```python
from build123d import *

# Parameters (mm, degrees)
BOSS_EXTRUDE1_DEPTH = 1.5
BOSS_EXTRUDE2_DEPTH = 3


with BuildPart() as part:
    # Sketch3 → Boss-Extrude1 (new body)
    with BuildSketch(Plane.XY):
        with BuildLine():
            Line((-20, 0), (-20, -97))
            ThreePointArc((-20, -97), (0, -117), (20, -97))
            Line((20, -97), (20, 0))
            ThreePointArc((20, 0), (0, 20), (-20, 0))
        make_face()
    extrude(amount=BOSS_EXTRUDE1_DEPTH)

    # Sketch5 → Boss-Extrude2 (add)
    with BuildSketch(Plane.XY.offset(1.5)):
        with BuildLine():
            Line((-19, 0), (-19, -97))
            ThreePointArc((-19, -97), (0, -116), (19, -97))
            Line((19, -97), (19, 0))
            ThreePointArc((19, 0), (0, 19), (-19, 0))
        make_face()
        with BuildLine():
            Line((-18, 0), (-18, -97))
            ThreePointArc((-18, -97), (0, -115), (18, -97))
            Line((18, -97), (18, 0))
            ThreePointArc((18, 0), (0, 18), (-18, 0))
        make_face(mode=Mode.SUBTRACT)
    extrude(amount=BOSS_EXTRUDE2_DEPTH)


solid = part.part
```
Work out the finished part from the listing and answer in its coordinate system (mm). A direction names the side the tool comes from. Coordinates: 2 decimals unless noted, no trailing zeros. Loops run counter-clockwise (first coordinate to the right, second up) from the corner with the lowest first, then second, coordinate; pieces in that order, holes last.
1) Section C-C (x = -14) is taken. Give the vertices of the cut face in (y, z).
Results:
outline: (-111.28, 0) - (14.28, 0) - (14.28, 1.5) - (12.85, 1.5) - (12.85, 4.5) - (11.31, 4.5) - (11.31, 1.5) - (-108.31, 1.5) - (-108.31, 4.5) - (-109.85, 4.5) - (-109.85, 1.5) - (-111.28, 1.5) - close
2) Section A-A (y = -91.5) is taken. Give the vertices of the cut face in (x, z).
Results:
outline: (-20, 0) - (20, 0) - (20, 1.5) - (19, 1.5) - (19, 4.5) - (18, 4.5) - (18, 1.5) - (-18, 1.5) - (-18, 4.5) - (-19, 4.5) - (-19, 1.5) - (-20, 1.5) - close
3) Flat-ended cylindrical pins translate along their axes: pin 1 (0.9 mm diameter, centred on y = -40.5, z = 3.5, fed in from +X); pin 2 (18 mm diameter, centred on x = -4, y = -80, fed in from +Z); pin 3 (1.5 mm diameter, centred on y = -38, z = 3, fed in from -X); pin 4 (8 mm diameter, centred on x = 0.5, y = -26.5, fed in from -Z). Find the tip coordinate at first contact, or state that the pin passes through.
Results:
pin 1: stops at x = 19
pin 2: stops at z = 1.5
pin 3: stops at x = -19
pin 4: stops at z = 0
4) For faces 1 (the flat face through (-18.4, -48.2, 4.5)), 2 (the flat face through (-18, -48, 3)), 3 (the flat face through (19, -49, 3)), 4 (the cylindrical face through (0, 19, 3)), 5 (the flat face through (-19, -48, 3)), determine the directions among +Z, -Z, +X, -X, +Y, -Y from which every point of the face is accessible in a straight line to the end or side of a thin tool.
Results:
face 1: +Z, +X, -X, +Y, -Y
face 2: +Z
face 3: +Z, +X, +Y, -Y
face 4: +Z, +Y
face 5: +Z, -X, +Y, -Y
5) Section B-B (z = 2.85) is taken. Give the vertices of the cut face in (x, y).
Results:
outline: (-19, -97) arc R19 ccw to (19, -97) - (19, 0) arc R19 ccw to (-19, 0) - close; hole (-18, -97) arc R18 ccw to (18, -97) - (18, 0) arc R18 ccw to (-18, 0) - close
6) For a pull along Y with two mould halves and no side action, classify faces 6 (the flat face through (0, -48, 1.5)), 7 (the flat face through (19.2, -48.2, 1.5)), 8 (the cylindrical face through (0, -116, 3)) as +Y half, -Y half, draft (parallel to the pull), parting line (faces both ways), or undercut.
Results:
face 6: undercut
face 7: draft
face 8: -Y half
7) Consider probe 1 along Y at (x, z) = (-0.5, 2.1); probe 2 along X at (y, z) = (-91, 2.8); probe 3 along Z at (x, y) = (-11.5, -74). Determine where each line is inside the solid, lowest interval first.
Results:
probe 1: y = -115.99 to -114.99, 17.99 to 18.99
probe 2: x = -19 to -18, 18 to 19
probe 3: z = 0 to 1.5
